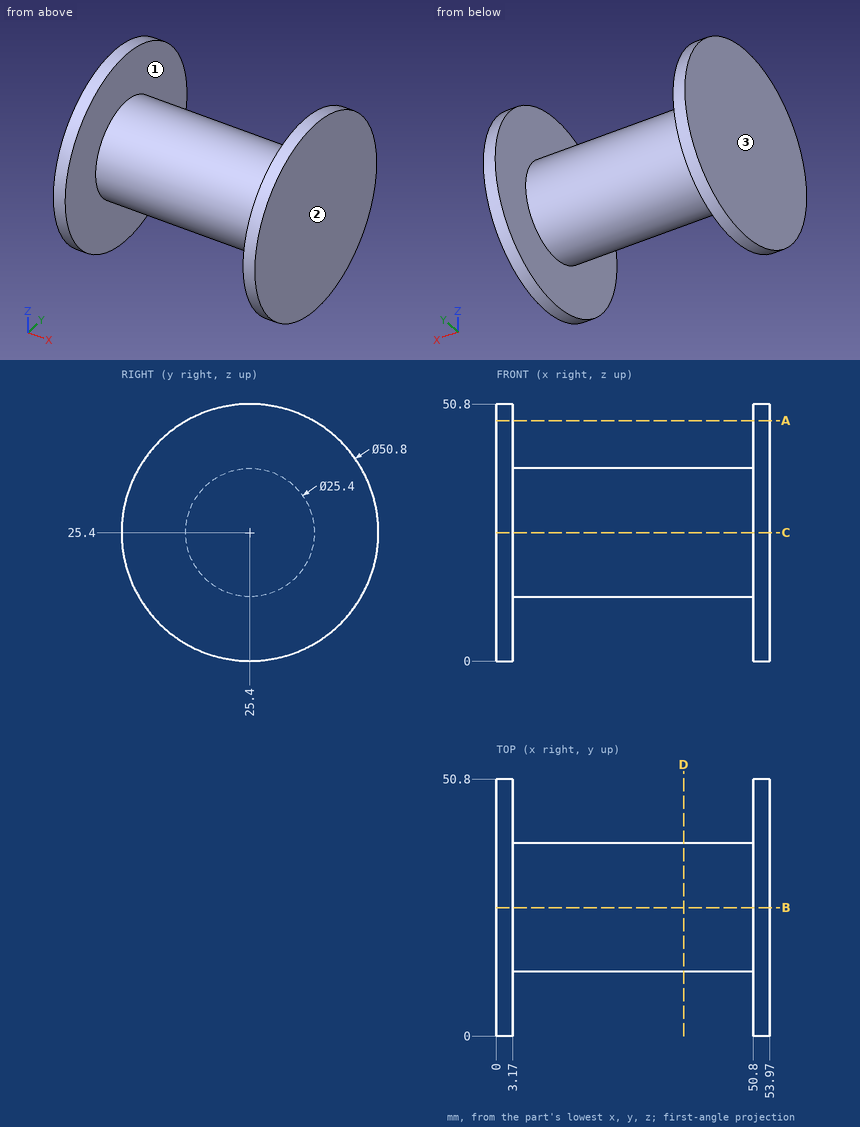
Study the drawing (mm; zero at the part's minimum x, y, z) and answer. Coordinates: 2 decimals unless noted, no trailing zeros. Loops run counter-clockwise (first coordinate to the right, second up) from the corner with the lowest first, then second, coordinate; pieces in that order, holes last. Notation, with made-up numbers: M 68,27.25 L 94,27.25 A25 cw 94,64.25 Z; hole C -16.75,-12 d6. An arc over 180 degrees is marked long. Answer in a Markdown table with one row per item. Add a question column.
1. Find section D-D, the plane x = 37. Write down the section's boundary in (y, z), then the cut area to 3 significant figures.
2. Flat-ended cylindrical pins translate along their axes: P1, Ø2, axis at x = 17.5, y = 29, coming from the +Z side; P2, Ø1.5, axis at x = 33.5, z = 32, coming from the -Y side; P3, Ø3, axis at x = 15, z = 9.5, coming from the -Y side; P4, Ø6, axis at x = 25, y = 11, coming from the +Z side. Find the tip coordinate at first contact, or state that the pin passes through.
3. Find section B-B, the plane y = 25.4. Write down the section's boundary in (x, z), then the cut area to 3 significant figures.
4. Consider L1, parallel to X at y = 36.5, z = 44; L2, parallel to Y at x = 50, z = 19; L3, parallel to Y at x = 51.5, z = 42.5. Determine where each line is inside the solid, lowest interval first.
5. Find section A-A, the plane z = 47.5. Write down the section's boundary in (x, y).
6. The mould has two halves that part along X. Classify the marked faces 1, 2 and 3: pulls with the +X half, pulls with the -X half, needs draft (parallel to the pull), parting line crosses it, or undercut.
Reported:
| question | item | result |
|---|---|---|
| 1 | outline | C 25.4,25.4 d25.4 |
| 1 | area | 507 mm^2 |
| 2 | P1 | stops at z = 37.83 |
| 2 | P2 | stops at y = 14.13 |
| 2 | P3 | passes through |
| 2 | P4 | stops at z = 31 |
| 3 | outline | M 0,0 L 3.17,0 L 3.17,12.7 L 50.8,12.7 L 50.8,0 L 53.97,0 L 53.97,50.8 L 50.8,50.8 L 50.8,38.1 L 3.17,38.1 L 3.17,50.8 L 0,50.8 Z |
| 3 | area | 1,530 mm^2 |
| 4 | L1 | x = 0 to 3.17, 50.8 to 53.97 |
| 4 | L2 | y = 14.43 to 36.37 |
| 4 | L3 | y = 6.62 to 44.18 |
| 5 | outline | M 0,12.88 L 3.17,12.88 L 3.17,37.92 L 0,37.92 Z; M 50.8,12.88 L 53.97,12.88 L 53.97,37.92 L 50.8,37.92 Z |
| 6 | face 1 | undercut |
| 6 | face 2 | pulls with the +X half |
| 6 | face 3 | pulls with the -X half |
